CAD build for the part. Positions are in the model's coordinates, mm. A direction names the side the tool comes from. Coordinates: 2 decimals unless noted, no trailing zeros. Loops run counter-clockwise (first coordinate to the right, second up) from the corner with the lowest first, then second, coordinate; pieces in that order, holes last.
1) Saw through at A-A, the plane z = 0. Write the cut outline in (x, y), and give its area (3 significant figures).
2) Saw through at C-C, the plane y = -2.5. Write the cut outline in (x, z), and give its area (3 significant figures).
3) Which spindle directions (+Z, -Z, +X, -X, +Y, -Y) get a long thin tool onto all of the face, cutting with end or side? Do faces 4 (the flat face through (23, 0, 0)), 5 (the flat face through (10, 1, 0)). Say none if no direction does.
4) Wall check: line 1 along Y through (x, z) = (6.5, 0); line 2 along X through (y, z) = (2.25, 1.75); line 3 along Y through (x, z) = (15.75, 7.5). Give the ranges that are in metal, low to high.
5) Saw through at D-D, the plane z = -4.25. Write the cut outline in (x, y).
6) Pin check, flat tips, straight feed: pin 1 Ø1.4 at (y, z) = (0.5, -1.5) entering from -X; pin 2 Ø10 at (x, y) = (16, 9.5) entering from +Z; pin 3 Ø2 at (x, z) = (12, 7) entering from +Y. Stop position of each tip, or through.
7) Saw through at B-B, the plane x = 15.75. Write the cut outline in (y, z), and give its area (3 significant figures).
8) Two-plate mould, pull along Z, no slides. Class faces 1 (the cylindrical face through (11.34, 0.53, 11.99)), 2 (the flat face through (5, -1, 0)), 3 (the flat face through (0, -2, 0)): +Z half, -Z half, draft (parallel to the pull), parting line (faces both ways), or undercut.
```python
from build123d import *

# Parameters (mm, degrees)
SKETCH1_R           = 12
BOSS_EXTRUDE1_DEPTH = 23
CUT_EXTRUDE1_DEPTH  = 10


with BuildPart() as part:
    # Sketch1 → Boss-Extrude1 (new body)
    with BuildSketch(Plane(origin=(0, 0, 0), x_dir=(0, 0, -1), z_dir=(1, 0, 0))):
        Circle(SKETCH1_R)
    extrude(amount=BOSS_EXTRUDE1_DEPTH)

    # Sketch2 → Cut-Extrude1 (cut)
    with BuildSketch(Plane.ZY):
        with BuildLine():
            ThreePointArc((3.5, 0), (-0.505293538, 3.463333429), (-3.354101966, -1))
            Line((-3.354101966, -1), (3.354101966, -1))
            ThreePointArc((3.354101966, -1), (3.463333429, -0.505293538), (3.5, 0))
        make_face()
    extrude(amount=-CUT_EXTRUDE1_DEPTH, mode=Mode.SUBTRACT)


solid = part.part
```
Data:
1. outline: (0, -12) - (23, -12) - (23, 12) - (0, 12) - (0, 3.5) - (10, 3.5) - (10, -1) - (0, -1) - close
1. area: 507 mm2
2. outline: (0, -11.74) - (23, -11.74) - (23, 11.74) - (0, 11.74) - close
2. area: 540 mm2
3. face 4: +Z, -Z, +X, +Y, -Y
3. face 5: -X
4. line 1: y = -12 to -1, 3.5 to 12
4. line 2: x = 10 to 23
4. line 3: y = -9.37 to 9.37
5. outline: (0, -11.22) - (23, -11.22) - (23, 11.22) - (0, 11.22) - close
6. pin 1: stops at x = 10
6. pin 2: stops at z = 11.12
6. pin 3: stops at y = 10.39
7. outline: circle Ø24 at (0, 0)
7. area: 452 mm2
8. face 1: parting line
8. face 2: undercut
8. face 3: draft
